Part model, mm, in its own coordinate system. A direction names the side the tool comes from. Coordinates: 2 decimals unless noted, no trailing zeros. Loops run counter-clockwise (first coordinate to the right, second up) from the corner with the lowest first, then second, coordinate; pieces in that order, holes last. Notation, with made-up numbers: (46, -37.75) -> (64, -37.75) arc R20 ccw to (64, -22.75) -> close; hole circle Ø2 at (25.25, 87). An arc over 180 degrees is marked (long way). Use one line per item in the form item = value. Start each with the question number.
(1) Mould opens along X. For faces 1 (the cylindrical face through (-85.96, -88.03, 4.93)), 2 (the cylindrical face through (-85.962, -34.497, 4.93)), 3 (the flat face through (-90, -29, 5)), 4 (the flat face through (-31, 30, 5)) say: +X half, -X half, draft (parallel to the pull), parting line (faces both ways), or undercut.
(2) 3-axis set-ups, long thin cutter, end or side, ignore diameter. For faces 5 (the flat face through (-25, 0, 5)), 6 (the flat face through (-30, -25, 0)): which of +Z, -Z, +X, -X, +Y, -Y reach the whole face in a straight line?
(3) Band-saw the part on C-C on y = -62.5. Give the cut face in (x, z).
(4) Band-saw the part on A-A on x = -60. Give the cut face in (y, z), then the cut area to 3 significant figures.
(5) Drill centre lines: L1, parallel to X at y = -2.5, z = 9.25; L2, parallel to X at y = -49, z = 7.5. Where is each one in solid material? Low to high. Write a range as [from, to].
(6) Band-saw the part on D-D on z = 3. Count the separate pieces of the cut face and the enclosed holes in it, then the cut area to 3 significant figures.
Autodesk Inventor part; units mm, degrees
ref_plane "YZ Plane" through (0, 0, 0) normal (1, 0, 0) x (0, 1, 0)
ref_plane "XZ Plane" through (0, 0, 0) normal (0, 1, 0) x (-1, 0, 0)
ref_plane "XY Plane" through (0, 0, 0) normal (0, 0, 1) x (1, 0, 0)
sketch "Sketch1" plane through (0, 0, 0) normal (0, 0, 1) x (1, 0, 0)
  line L0 (-79, -35) -> (19, -35)
  line L1 (25, -41) -> (25, -79)
  line L2 (30, -32) -> (30, -36)
  line L3 (30, -24) -> (30, -28)
  line L4 (28, -30) -> (24, -30)
  line L5 (-24, -30) -> (-28, -30)
  line L6 (-30, -28) -> (-30, -24)
  line L7 (-88, -30) -> (-84, -30)
  line L8 (-85, -79) -> (-85, -41)
  line L9 (19, -85) -> (-79, -85)
  line L10 (30, -84) -> (30, -88)
  line L11 (24, -90) -> (19, -85)
  line L12 (28, -90) -> (24, -90)
  line L13 (-84, -90) -> (-88, -90)
  line L14 (-90, -88) -> (-90, -84)
  line L15 (-30, 24) -> (-30, 28)
  line L16 (-28, 30) -> (-24, 30)
  line L17 (24, 30) -> (28, 30)
  line L18 (30, 28) -> (30, 24)
  line L19 (25, 19) -> (25, -19)
  line L20 (-25, -19) -> (-25, 19)
  line L21 (19, -25) -> (-19, -25)
  line L22 (-19, 25) -> (19, 25)
  line L23 (25, 25) -> (-25, 25)
  line L24 (-25, 25) -> (-25, -25)
  line L25 (-25, -25) -> (25, -25)
  line L26 (25, -25) -> (25, 25)
  line L27 (25, -35) -> (-85, -35)
  line L28 (-85, -35) -> (-85, -85)
  line L29 (-85, -85) -> (25, -85)
  line L30 (25, -85) -> (25, -35)
  line L31 (30, -30) -> (-90, -30)
  line L32 (-90, -30) -> (-90, -90)
  line L33 (-90, -90) -> (30, -90)
  line L34 (30, -90) -> (30, -30)
  line L35 (30, 30) -> (-30, 30)
  line L36 (-30, 30) -> (-30, -30)
  line L37 (-30, -30) -> (30, -30)
  line L38 (30, -30) -> (30, 30)
  line L39 (-30, -30) -> (-90, -30)
  line L40 (-90, -30) -> (-90, 30)
  line L41 (-90, 30) -> (-30, 30)
  line L42 (-30, 30) -> (-30, -30)
  line L43 (-30, -25) -> (-35, -25)
  line L44 (-35, -25) -> (-85, -25)
  line L45 (-85, -25) -> (-85, 25)
  line L46 (-85, 25) -> (-35, 25)
  line L47 (-35, 25) -> (-35, -25)
  circle A0 centre (-26.7678, 26.7678) radius 1.5
  circle A1 centre (26.7678, 26.7678) radius 1.5
  circle A2 centre (26.7678, -26.7678) radius 1.5
  circle A3 centre (-26.7678, -26.7678) radius 1.5
  circle A4 centre (26.768, -33.232) radius 1.5
  circle A5 centre (26.768, -86.768) radius 1.5
  circle A6 centre (-86.768, -86.768) radius 1.5
  circle A7 centre (-86.768, -33.232) radius 1.5
  circle A8 centre (-33.2322, 26.7678) radius 1.5
  circle A9 centre (-86.7678, 26.7678) radius 1.5
  circle A10 centre (-86.7678, -26.7678) radius 1.5
  circle A11 centre (-33.2322, -26.7678) radius 1.5
  point P0 (0, 0)
  dimension "d0" = 5
extrude "Extrusion1" add sketch "Sketch1" along normal blind 10
fillet "Fillet1" radius 2 4 edges at (-90, 30, 5) (-90, -90, 5) (30, -90, 5) (30, 30, 5)
properties part number "frame_demo_2x2_xyxx"
A:
q1.face_1 = undercut
q1.face_2 = undercut
q1.face_3 = -X half
q1.face_4 = draft
q2.face_5 = +Z, -Z
q2.face_6 = -Z, +X, -X, +Y, -Y
q3.outline = (-90, 0) -> (-85, 0) -> (-85, 10) -> (-90, 10) -> close; (25, 0) -> (30, 0) -> (30, 10) -> (25, 10) -> close
q4.outline = (-90, 0) -> (-85, 0) -> (-85, 10) -> (-90, 10) -> close; (-35, 0) -> (-25, 0) -> (-25, 10) -> (-35, 10) -> close; (25, 0) -> (30, 0) -> (30, 10) -> (25, 10) -> close
q4.area = 200 mm²
q5.L1 = [-90, -85], [-35, -25], [25, 30]
q5.L2 = [-90, -85], [25, 30]
q6.separate_pieces = 1
q6.enclosed_holes = 15
q6.area = 3,810 mm²
